Input: part model. Units: mm. Frame: model coordinates. Face numbers are marked on the shaded views. A direction names the side the tool comes from. Coordinates: 2 decimals unless noted, no trailing zeros. Loops run counter-clockwise (first coordinate to the right, second up) from the corner with the lowest first, then second, coordinate; pieces in that order, holes last.
Item 1: Section D-D on z = 11.5. Return loops of the section in (x, y).
Item 2: Section B-B on y = 2.7. Return loops of the section in (x, z) (3 decimals).
Item 3: Section C-C on x = -10. Return loops of the section in (y, z) (3 decimals), and give its area (3 significant figures).
Item 4: Ray query, line 1 along X through (y, z) = (2.25, 0) (3 decimals); line 2 along Z through (x, y) = (-10, 2.35) (3 decimals); line 3 along Z through (x, y) = (9.75, 1.95). Return the intervals inside material, ascending.
Item 5: Contact query for flat-ended pins moving along their axis: P1, Ø2.5, axis at y = 2.5, z = 13.5, coming from the -X side; P2, Ø2.5, axis at y = 4, z = 16.5, coming from the +X side; P3, Ø1.6, axis at x = -8.5, y = 4, coming from the +Z side. Output: stop coordinate, or through.
Item 6: Section A-A on z = 0. Return loops of the section in (x, y) (3 decimals), and give its area (3 significant figures).
Item 7: Pull-direction query (Z, two-part tool) for the marked faces 1, 2 and 3; classes: released by +Z, released by -Z, zero draft, split by the parting line, or undercut.
Item 8: Reachability of the marked faces 4, 5 and 6 from +Z, -Z, +X, -X, +Y, -Y: full face, straight path, thin tool, end or side. Return the list, or none.
```python
from build123d import *

# Parameters (mm, degrees)
SKETCH1_R           = 1.325
BOSS_EXTRUDE1_DEPTH = 5.4
CHAMFER2_SIZE       = 0.25
FILLET4_START       = -1
FILLET4_DEPTH       = 7
FILLET4_2_DEPTH     = 5.4
FILLET5_R           = 1.5


with BuildPart() as part:
    # Sketch1 → Boss-Extrude1 (new body)
    with BuildSketch(Plane(origin=(0, 0, 0), x_dir=(1, 0, 0), z_dir=(0, 1, 0))):
        with BuildLine():
            Line((-6, -7.75), (-6, -21.25))
            Line((-6, -21.25), (6, -21.25))
            Line((6, -21.25), (6, -7.75))
            Line((6, -7.75), (7.5, -7.75))
            Line((7.5, -7.75), (7.5, -4.25))
            Line((7.5, -4.25), (9, -4.25))
            ThreePointArc((9, -4.25), (13.25, 0), (9, 4.25))
            Line((9, 4.25), (-9, 4.25))
            ThreePointArc((-9, 4.25), (-13.25, 0), (-9, -4.25))
            Line((-9, -4.25), (-7.5, -4.25))
            Line((-7.5, -4.25), (-7.5, -7.75))
            Line((-7.5, -7.75), (-6, -7.75))
        make_face()
        with Locations(Location((-10, 0, 0), (0, 0, 90))):
            Circle(SKETCH1_R, mode=Mode.SUBTRACT)
        with Locations(Location((10, 0, 0), (0, 0, 90))):
            Circle(SKETCH1_R, mode=Mode.SUBTRACT)
    extrude(amount=BOSS_EXTRUDE1_DEPTH)

    # Chamfer2
    chamfer2_edges = [part.edges().sort_by_distance(p)[0] for p in [
        (-10, 0, 1.325),
        (-10, 5.4, 1.325),
        (10, 0, 1.325),
        (10, 5.4, 1.325),
    ]]
    chamfer(chamfer2_edges, length=CHAMFER2_SIZE)

    # Fillet4: read off the stored shape, not the designer's step
    # Fillet4 outline → Fillet4 (cut)
    with BuildSketch(Plane(origin=(0, 0, 0), x_dir=(1, 0, 0), z_dir=(0, 1, 0)).offset(FILLET4_START)):
        with BuildLine():
            ThreePointArc((6, -19.75), (5.560660172, -20.810660172), (4.5, -21.25))
            Line((4.5, -21.25), (6, -21.25))
            Line((6, -21.25), (6, -19.75))
        make_face()
        with BuildLine():
            ThreePointArc((-4.5, -21.25), (-5.560660172, -20.810660172), (-6, -19.75))
            Line((-6, -19.75), (-6, -21.25))
            Line((-6, -21.25), (-4.5, -21.25))
        make_face()
    extrude(amount=FILLET4_DEPTH, mode=Mode.SUBTRACT)

    # Fillet4 2 outline → Fillet4 2 (add)
    with BuildSketch(Plane(origin=(0, 0, 0), x_dir=(1, 0, 0), z_dir=(0, 1, 0))):
        with BuildLine():
            Line((6, -7.75), (6, -9.25))
            ThreePointArc((6, -9.25), (6.439339828, -8.189339828), (7.5, -7.75))
            Line((7.5, -7.75), (6, -7.75))
        make_face()
        with BuildLine():
            ThreePointArc((-7.5, -7.75), (-6.439339828, -8.189339828), (-6, -9.25))
            Line((-6, -9.25), (-6, -7.75))
            Line((-6, -7.75), (-7.5, -7.75))
        make_face()
    extrude(amount=FILLET4_2_DEPTH)

    # Fillet5
    fillet5_edges = [part.edges().sort_by_distance(p)[0] for p in [
        (7.5, 2.7, 7.75),
        (-7.5, 2.7, 7.75),
    ]]
    fillet(fillet5_edges, radius=FILLET5_R)


solid = part.part
```
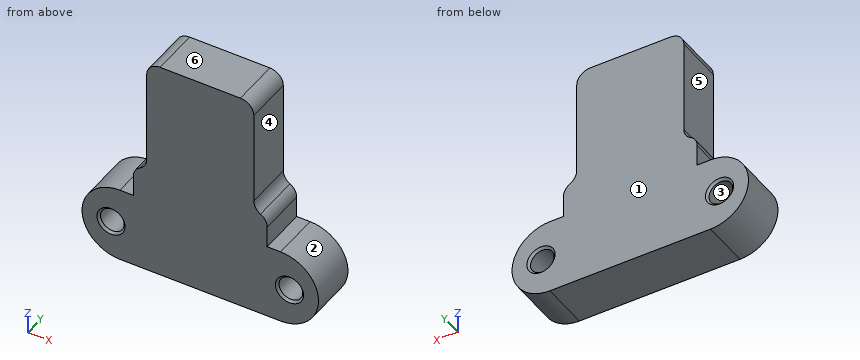
Results found:
1. outline: (-6, 0) - (6, 0) - (6, 5.4) - (-6, 5.4) - close
2. outline: (-9, -4.25) - (9, -4.25) arc R4.25 ccw to (9, 4.25) - (7.5, 4.25) - (7.5, 6.652) arc R1.5 ccw to (6.75, 7.951) arc R1.5 cw to (6, 9.25) - (6, 19.75) arc R1.5 ccw to (4.5, 21.25) - (-4.5, 21.25) arc R1.5 ccw to (-6, 19.75) - (-6, 9.25) arc R1.5 cw to (-6.75, 7.951) arc R1.5 ccw to (-7.5, 6.652) - (-7.5, 4.25) - (-9, 4.25) arc R4.25 ccw to start; hole circle Ø2.65 at (-10, 0); hole circle Ø2.65 at (10, 0)
3. outline: (0, -4.131) - (5.4, -4.131) - (5.4, -1.575) - (5.15, -1.325) - (0.25, -1.325) - (0, -1.575) - close; (0, 1.575) - (0.25, 1.325) - (5.15, 1.325) - (5.4, 1.575) - (5.4, 4.131) - (0, 4.131) - close
3. area: 30.2 mm2
4. line 1: x = -13.25 to -11.325, -8.675 to 8.675, 11.325 to 13.25
4. line 2: z = -4.131 to -1.325, 1.325 to 4.131
4. line 3: z = -4.18 to -1.3, 1.3 to 4.18
5. P1: stops at x = -6
5. P2: stops at x = 6
5. P3: stops at z = 4.25
6. outline: (-13.25, 0) - (-11.575, 0) - (-11.325, 0.25) - (-11.325, 5.15) - (-11.575, 5.4) - (-13.25, 5.4) - close; (-8.675, 0.25) - (-8.425, 0) - (8.425, 0) - (8.675, 0.25) - (8.675, 5.15) - (8.425, 5.4) - (-8.425, 5.4) - (-8.675, 5.15) - close; (11.325, 0.25) - (11.575, 0) - (13.25, 0) - (13.25, 5.4) - (11.575, 5.4) - (11.325, 5.15) - close
6. area: 114 mm2
7. face 1: zero draft
7. face 2: split by the parting line
7. face 3: undercut
8. face 4: +Z, +X, +Y, -Y
8. face 5: +Z, -X, +Y, -Y
8. face 6: +Z, +X, -X, +Y, -Y
